Autodesk Inventor part; units mm, degrees
ref_plane "YZ Plane" through (0, 0, 0) normal (1, 0, 0) x (0, 1, 0)
ref_plane "XZ Plane" through (0, 0, 0) normal (0, 1, 0) x (-1, 0, 0)
ref_plane "XY Plane" through (0, 0, 0) normal (0, 0, 1) x (1, 0, 0)
sketch "Sketch1" plane through (0, 0, 0) normal (0, 0, 1) x (1, 0, 0)
  line L0 (10, 10) -> (-10, 10) construction
  line L1 (-10, 10) -> (-10, -10) construction
  line L2 (-10, -10) -> (10, -10) construction
  line L3 (10, -10) -> (10, 10) construction
  line L4 (-7, -7) -> (-7, 7) construction
  line L5 (-7, 7) -> (7, 7) construction
  line L6 (7, 7) -> (7, -7) construction
  line L7 (7, -7) -> (-7, -7) construction
  line L8 (13.5, 13.5) -> (-13.5, 13.5)
  line L9 (-13.5, 13.5) -> (-13.5, -13.5)
  line L10 (-13.5, -13.5) -> (13.5, -13.5)
  line L11 (13.5, -13.5) -> (13.5, 13.5)
  line L12 (10.5, 10.5) -> (-10.5, 10.5)
  line L13 (-10.5, 10.5) -> (-10.5, -10.5)
  line L14 (-10.5, -10.5) -> (10.5, -10.5)
  line L15 (10.5, -10.5) -> (10.5, 10.5)
  point P0 (0, 0)
  point P1 (-10.5, 0)
  point P2 (0, 10.5)
  dimension "d36" = 21
  dimension "d37" = 21
  dimension "d38" = 3
  dimension "d39" = 3
  dimension "d40" = 3
  dimension "d41" = 3
extrude "Extrusion1" add sketch "Sketch1" against normal blind 55
sketch "Sketch2" plane through (-13.5, -13.5, 0) normal (-1, 0, 0) x (0, 0, 1)
  line L0 (-80.4804, 19) -> (40.5, 19)
  line L1 (40.5, 19) -> (40.5, 9)
  line L2 (40.5, 9) -> (-80.4804, 9)
  line L3 (-80.4804, 9) -> (-80.4804, 19)
  line L4 (0, 27) -> (-55, 27)
  point P0 (0, 13.5)
  dimension "d7" = 10
  dimension "d8" = 8
extrude "Extrusion2" cut sketch "Sketch2" against normal blind 15.3125
sketch "Sketch3" plane through (-13.5, 13.5, 0) normal (0, 1, 0) x (1, 0, 0)
  line L0 (27, 0) -> (0, 0)
  line L1 (3, 55) -> (23, 55)
  line L2 (27, 0) -> (22, 0)
  line L3 (22, 0) -> (22, 55)
  line L4 (22, 55) -> (27, 55)
  line L5 (27, 55) -> (27, 0)
  point P0 (13.5, 0)
  dimension "d11" = 5
extrude "Extrusion3" add sketch "Sketch3" along normal blind 42.3
sketch "Sketch4" plane through (13.5, -13.5, 0) normal (1, 0, 0) x (0, 0, -1)
  line L0 (0, 27) -> (55, 27)
  circle A0 centre (27.5, 46) radius 18
  line L1 (0, 69.3) -> (55, 69.3)
  circle A1 centre (27.5, 46) radius 3
  point P0 (0, 13.5)
  point P1 (27.5, 69.3)
  dimension "d14" = 36
  dimension "d15" = 19
  dimension "d16" = 6
extrude "Extrusion4" cut sketch "Sketch4" against normal blind 42.3 contours A1
sketch "Sketch5" plane through (13.5, -13.5, 0) normal (1, 0, 0) x (0, 0, -1)
  circle A0 centre (27.5, 46) radius 3
  circle A1 centre (27.5, 46) radius 10.5
  point P0 (0, 13.5)
  dimension "d19" = 21
extrude "Extrusion5" cut sketch "Sketch5" against normal blind 42.3
sketch "Sketch6" plane through (13.5, -13.5, 0) normal (1, 0, 0) x (0, 0, -1)
  circle A0 centre (27.5, 30.5) radius 1.5
  circle A1 centre (19.1831, 33.1223) radius 1.495
  circle A2 centre (14.9426, 52.25) radius 1.5
  circle A3 centre (21.372, 58.1415) radius 1.495
  circle A4 centre (40.0574, 52.25) radius 1.5
  circle A5 centre (41.9448, 43.7362) radius 1.495
  point P0 (0, 13.5)
extrude "Extrusion6" cut sketch "Sketch6" against normal blind 42.3
sketch "Sketch7" plane through (13.5, -13.5, 0) normal (1, 0, 0) x (0, 0, -1)
  circle A0 centre (10, 13.5) radius 1.5
  circle A1 centre (45, 13.5) radius 1.5
  line L0 (0, 0) -> (0, 69.3)
  line L1 (55, 0) -> (55, 69.3)
  point P0 (0, 13.5)
  dimension "d24" = 3
  dimension "d25" = 3
  dimension "d26" = 10
  dimension "d27" = 10
extrude "Extrusion7" cut sketch "Sketch7" against normal blind 10
sketch "Sketch8" plane through (-13.5, -13.5, 0) normal (0, -1, 0) x (1, 0, 0)
  circle A0 centre (13.5, -10) radius 1.5
  circle A1 centre (13.5, -45) radius 1.5
  line L0 (27, -55) -> (0, -55)
  line L1 (0, 0) -> (27, 0)
  point P0 (13.5, 0)
  point P1 (13.5, 0)
  point P2 (13.5, 0)
  dimension "d30" = 3
  dimension "d31" = 3
  dimension "d32" = 10
  dimension "d33" = 10
extrude "Extrusion8" cut sketch "Sketch8" against normal through all
properties part number "enc holder"
For this review, take the finished solid that the model builds, in its own axes (mm). A direction names the side the tool comes from. Give positions to 0.01 mm unless a question says otherwise; leave off trailing zeros. Order: outer loops, then holes, each group sorted by start corner. A loop starts at its lowest first (then second) coordinate and runs counter-clockwise, first axis right, second up. Notation, with made-up numbers: (-3, 55.25) - (14, 55.25) arc R18 ccw to (14, 70.25) - close; hole circle Ø3 at (-33, -34). An arc over 180 degrees is marked (long way). Answer as a JSON object with one key per item and string values. Group by question number.
Item 1: Take a section at B-B on y = 32.5. Give the boundary of the cut face in (x, z).
Item 2: Take a section at C-C on z = -10. Give the boundary of the cut face in (x, y), and give its area (4 significant figures).
Item 3: Machinability: for faces 4 (the flat face through (0, 10.5, -27)), 5 (the flat face through (-12, -4.5, -27)), 6 (the flat face through (8.5, 44, -27)), which of the approach directions +Z, -Z, +X, -X, +Y, -Y give a long, thin tool a straight path to every point of the face, cutting with its end or side? Answer none if there is none.
Item 4: Clearance check with flat-ended pins moving along their axes: pin 1 Ø6 at (x, z) = (-6.5, -14) entering from +Y; pin 2 Ø5 at (y, z) = (0, -10) entering from -X; pin 3 Ø4 at (y, z) = (19.62, -19.18) entering from -X; pin 4 Ø2.5 at (y, z) = (44.64, -21.37) entering from -X. State where each tip first meets the part, or that it passes through.
Item 5: Take a section at A-A on x = -5. Give the boundary of the cut face in (y, z).
Item 6: Take a section at D-D on x = 0. Give the boundary of the cut face in (y, z), and give its area (3 significant figures).
Item 7: Draft analysis for pull direction Z (two halves, no side actions). For faces 1 (the flat face through (10.5, 0, -27)), 2 (the cylindrical face through (-0.325, -12.021, -46.464)), 3 (the flat face through (4, 13, 0)), state which applies: pulls with the +Z half, pulls with the -Z half, needs draft (parallel to the pull), parting line crosses it, or undercut.
Item 8: Wall thickness on line 1 along Z through (x, y) = (0, 12.65); line 2 along Y through (x, z) = (3.75, -42); line 3 along X through (y, z) = (28.5, -11.5): over which ranges is each line inside the solid? List them lowest first.
Reported:
{
 "1": {"outline": "(8.5, -55) - (13.5, -55) - (13.5, -38) - (8.5, -38) - close; (8.5, -17) - (13.5, -17) - (13.5, 0) - (8.5, 0) - close"},
 "2": {"outline": "(-13.5, -13.5) - (-1.5, -13.5) - (-1.5, -10.5) - (-10.5, -10.5) - (-10.5, -4.5) - (-13.5, -4.5) - close; (-13.5, 5.5) - (-10.5, 5.5) - (-10.5, 10.5) - (-1.5, 10.5) - (-1.5, 13.5) - (-13.5, 13.5) - close; (1.5, -13.5) - (13.5, -13.5) - (13.5, -1.5) - (10.5, -1.5) - (10.5, -10.5) - (1.5, -10.5) - close; (1.5, 10.5) - (10.5, 10.5) - (10.5, 1.5) - (13.5, 1.5) - (13.5, 55.8) - (8.5, 55.8) - (8.5, 13.5) - (1.5, 13.5) - close", "area": "442.5 mm^2"},
 "3": {"face 4": "+Z, -Z", "face 5": "+Z, -Z, -X", "face 6": "+Z, -Z, -X, +Y"},
 "4": {"pin 1": "y = 13.5", "pin 2": "x = 10.5", "pin 3": "x = 8.5", "pin 4": "through"},
 "5": {"outline": "(-13.5, -55) - (-10.5, -55) - (-10.5, 0) - (-13.5, 0) - close; (10.5, -55) - (13.5, -55) - (13.5, 0) - (10.5, 0) - close"},
 "6": {"outline": "(-13.5, -55) - (-10.5, -55) - (-10.5, -46.5) - (-13.5, -46.5) - close; (-13.5, -43.5) - (-10.5, -43.5) - (-10.5, -11.5) - (-13.5, -11.5) - close; (-13.5, -8.5) - (-10.5, -8.5) - (-10.5, 0) - (-13.5, 0) - close; (10.5, -55) - (13.5, -55) - (13.5, -46.5) - (10.5, -46.5) - close; (10.5, -43.5) - (13.5, -43.5) - (13.5, -11.5) - (10.5, -11.5) - close; (10.5, -8.5) - (13.5, -8.5) - (13.5, 0) - (10.5, 0) - close", "area": "294 mm^2"},
 "7": {"face 1": "needs draft", "face 2": "undercut", "face 3": "pulls with the +Z half"},
 "8": {"line 1": "-55 to -46.5, -43.5 to -11.5, -8.5 to 0", "line 2": "-13.5 to -10.5, 10.5 to 13.5", "line 3": "8.5 to 13.5"}
}
